```python
from build123d import *

# Parameters (mm, degrees)
EXTRUSION1_DEPTH        = 7.5
ESQUISSE2_R             = 2
EXTRUSION2_DEPTH        = 9
ESQUISSE3_R             = 2
ENL_V_MAT_EXTRU_1_DEPTH = 9


with BuildPart() as part:
    # Esquisse1 → Extrusion1 (new, symmetric)
    with BuildSketch(Plane(origin=(0, 0, 0), x_dir=(1, 0, 0), z_dir=(0, 1, 0))):
        Polygon((-1.449747468, 3.5), (1.449747468, 3.5), (3.5, 1.449747468), (3.5, -1.449747468), (1.449747468, -3.5), (-1.449747468, -3.5), (-3.5, -1.449747468), (-3.5, 1.449747468), align=None)
    extrude(amount=EXTRUSION1_DEPTH, both=True)

    # Esquisse2 → Extrusion2 (add)
    with BuildSketch(Plane(origin=(0, 7.5, 0), x_dir=(1, 0, 0), z_dir=(0, 1, 0))):
        with Locations(Location((0, 0, 0), (0, 0, 270))):
            Circle(ESQUISSE2_R)
    extrude(amount=EXTRUSION2_DEPTH)

    # Esquisse3 → Enlèv. mat.-Extru.1 (cut)
    with BuildSketch(Plane.XZ.offset(7.5)):
        with Locations(Location((0, 0, 0), (0, 0, 90))):
            Circle(ESQUISSE3_R)
    extrude(amount=-ENL_V_MAT_EXTRU_1_DEPTH, mode=Mode.SUBTRACT)


solid = part.part
```
Geometry: final body of the model. Coordinates: model frame, mm. A direction names the side the tool comes from. Round coordinates to 2 decimals unless told otherwise and drop trailing zeros. Write each loop counter-clockwise with the first axis right and the second up, starting at its lowest first coordinate (ties: lowest second). Pieces come first, ordered by that corner, then holes. Notation, with made-up numbers: M -23.75,50 L -16.75,50 A19 cw -16.75,56 Z; hole C 77.5,26.5 d1. An arc over 180 degrees is marked long. Answer in a Markdown table with one row per item. Add a question column.
(1) Contact query for flat-ended pins moving along their axis: pin 1 (1.5 mm diameter, centred on y = 13, z = 2, fed in from -X); pin 2 (1.5 mm diameter, centred on x = 2.5, z = 2, fed in from +Y); pin 3 (4 mm diameter, centred on x = 1.5, z = 0, fed in from -Y); pin 4 (4 mm diameter, centred on x = 1.5, y = 13, fed in from +Z). Output: stop coordinate, or through.
(2) Cut plane A-A, the plane y = 4. Return the cut outline in (x, z), then the cut area to 3 significant figures.
(3) Cut plane B-B, the plane x = 0. Return the cut outline in (y, z), then the cut area to 3 significant figures.
(4) Cut plane D-D, the plane z = 0.25. Return the cut outline in (x, y).
(5) Ray query, L1, parallel to X at y = -5, z = 0; L2, parallel to Y at x = 1.75, z = -2.25; L3, parallel to Y at x = 1.25, z = 0. Return the intervals inside material, ascending.
(6) Cut plane C-C, the plane y = -0.5. Return the cut outline in (x, z), then the cut area to 3 significant figures.
(7) Reachability of faces 1 (the face through (-2, 7.5, -2)), 2 (the face through (0, 0, -3.5)), 3 (the face through (2, -3, 0)) from +Z, -Z, +X, -X, +Y, -Y: full face, straight path, thin tool, end or side. Return the list, or none.
(8) Draft query along X for faces 4 (the face through (-2, 12, 0)), 5 (the face through (0, 1.5, 0)), 6 (the face through (0, 16.5, 0)). Return one class per face: pulls with the +X half, pulls with the -X half, needs draft (parallel to the pull), parting line crosses it, or undercut.
Established:
| question | item | result |
|---|---|---|
| 1 | pin 1 | x = -1.56 |
| 1 | pin 2 | y = 7.5 |
| 1 | pin 3 | y = -7.5 |
| 1 | pin 4 | z = 2 |
| 2 | outline | M -3.5,-1.45 L -1.45,-3.5 L 1.45,-3.5 L 3.5,-1.45 L 3.5,1.45 L 1.45,3.5 L -1.45,3.5 L -3.5,1.45 Z |
| 2 | area | 40.6 mm² |
| 3 | outline | M -7.5,-3.5 L 7.5,-3.5 L 7.5,-2 L 16.5,-2 L 16.5,2 L 7.5,2 L 7.5,3.5 L -7.5,3.5 L -7.5,2 L 1.5,2 L 1.5,-2 L -7.5,-2 Z |
| 3 | area | 105 mm² |
| 4 | outline | M -3.5,-7.5 L -1.98,-7.5 L -1.98,1.5 L 1.98,1.5 L 1.98,-7.5 L 3.5,-7.5 L 3.5,7.5 L 1.98,7.5 L 1.98,16.5 L -1.98,16.5 L -1.98,7.5 L -3.5,7.5 Z |
| 5 | L1 | -3.5 to -2, 2 to 3.5 |
| 5 | L2 | -7.5 to 7.5 |
| 5 | L3 | 1.5 to 16.5 |
| 6 | outline | M -3.5,-1.45 L -1.45,-3.5 L 1.45,-3.5 L 3.5,-1.45 L 3.5,1.45 L 1.45,3.5 L -1.45,3.5 L -3.5,1.45 Z; hole C 0,0 d4 |
| 6 | area | 28.0 mm² |
| 7 | face 1 | +Y |
| 7 | face 2 | -Z, +X, -X, +Y, -Y |
| 7 | face 3 | -Y |
| 8 | face 4 | parting line crosses it |
| 8 | face 5 | undercut |
| 8 | face 6 | needs draft |
